Source: CAD feature listing. Evaluate the final solid. Frame: model axes, mm. Face numbers are marked on the shaded views. Give positions to 0.01 mm unless a question says otherwise; leave off trailing zeros. Loops run counter-clockwise (first coordinate to the right, second up) from the corner with the lowest first, then second, coordinate; pieces in that order, holes last. Notation, with made-up numbers: M 44.25,63 L 96.25,63 A21 cw 96.25,76 Z; hole C 21.25,28 d7. An arc over 180 degrees is marked long. Answer in a Markdown table with one row per item.
```python
from build123d import *

# Parameters (mm, degrees)
F0_R     = 12.5
F0_R_2   = 11
F1_DEPTH = 16
F3_DEPTH = 16
F4_DEPTH = 26
F6_DEPTH = 16


# Not quite as in the source:
# - a feature of the source that left no trace in its solid (it failed there, or was rolled back) is left out
# - a feature names something its author has since deleted; it is built from what else it names


with BuildPart() as f1:
    # F0 (on Front) → F1 (new body)
    with BuildSketch(Plane.XZ):
        Circle(F0_R)
        Circle(F0_R_2, mode=Mode.SUBTRACT)
    extrude(amount=F1_DEPTH)

    # F2 (on Front) → F3 (join)
    with BuildSketch(Plane.XZ):
        with BuildLine():
            Line((7.2098509409, 14.1820398122), (-7.7328206971, 14.1820398122))
            Line((-7.7328206971, 14.1820398122), (-7.7328206971, 9.7571304068))
            ThreePointArc((-7.7328206971, 9.7571304068), (0.3692249529, -12.210413225), (7.2098509409, 10.1820398122))
            Line((7.2098509409, 10.1820398122), (7.2098509409, 14.1820398122))
        make_face()
    extrude(amount=F3_DEPTH)

    # F0 (on Front) → F4 (cut)
    with BuildSketch(Plane.XZ):
        Circle(F0_R_2)
    extrude(amount=F4_DEPTH, mode=Mode.SUBTRACT)

    # F5 (on face) → F6 (join)
    with BuildSketch(Plane.XZ.offset(16)):
        with BuildLine():
            ThreePointArc((-7.7328206971, 14.1820398122), (-11.492539371, 7.5535946754), (-12.5, 0))
            ThreePointArc((-12.5, 0), (-11.2452269589, 5.4584677926), (-7.7328206971, 9.8210734681))
            Line((-7.7328206971, 9.8210734681), (-7.7328206971, 14.1820398122))
        make_face()
        with BuildLine():
            ThreePointArc((7.2098509409, 10.2111727735), (11.0989444715, 5.7500810098), (12.5, 0))
            ThreePointArc((12.5, 0), (11.2484098162, 7.6108139553), (7.2098509409, 14.1820398122))
            Line((7.2098509409, 14.1820398122), (7.2098509409, 10.2111727735))
        make_face()
    extrude(amount=-F6_DEPTH)


solid = f1.part
```
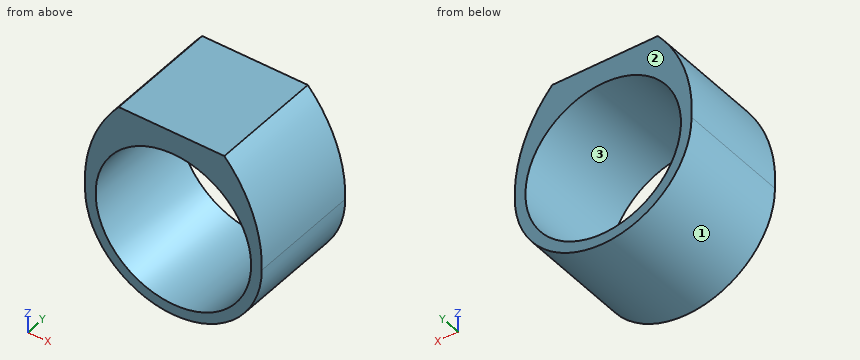
1) Section A-A, the plane x = 0. Return loops of the section in (y, z), then the cut area to 3 significant figures.
Reply:
| item | result |
|---|---|
| outline | M -16,-12.5 L 0,-12.5 L 0,-11 L -16,-11 Z; M -16,11 L 0,11 L 0,14.18 L -16,14.18 Z |
| area | 74.9 mm² |
2) Section B-B, the plane z = -9.75. Return loops of the section in (x, y), then the cut area to 3 significant figures.
Reply:
| item | result |
|---|---|
| outline | M -7.82,-16 L -5.09,-16 L -5.09,0 L -7.82,0 Z; M 5.09,-16 L 7.82,-16 L 7.82,0 L 5.09,0 Z |
| area | 87.3 mm² |
3) Pin query (flat end, axial travel): pin 1 Ø8 at (y, z) = (-4, 9.5) entering from +X. Return the tip coordinate at first contact, or that it passes through.
Reply:
| item | result |
|---|---|
| pin 1 | stops at x = 11.91 |
4) Pull-direction query (X, two-part tool) for the marked faces 1, 2 and 3; classes: released by +X, released by -X, zero draft, split by the parting line, or undercut.
Reply:
| item | result |
|---|---|
| face 1 | split by the parting line |
| face 2 | zero draft |
| face 3 | undercut |
5) Material intervals for L1, parallel to Z at x = 0, y = -10.25; L2, parallel to X at y = -6.75, z = -0.25; L3, parallel to Z at x = 8.75, y = -14, sorted ascending.
Reply:
| item | result |
|---|---|
| L1 | z = -12.5 to -11, 11 to 14.18 |
| L2 | x = -12.5 to -11, 11 to 12.5 |
| L3 | z = -8.93 to -6.67, 6.67 to 12.29 |
6) Section C-C, the plane y = -1.5. Return loops of the section in (x, z).
Reply:
| item | result |
|---|---|
| outline | M -12.5,0 A12.5 ccw 12.5,0 A20 ccw 7.21,14.18 L -7.73,14.18 A20 ccw Z; hole C 0,0 d22 |
